from build123d import *

# Parameters (mm, degrees)
SKETCH1_R                = 12.499992756
SKETCH1_R_2              = 4.5
BOSS_EXTRUDE1_DEPTH      = 10
BOSS_EXTRUDE2_DEPTH      = 11
BOSS_EXTRUDE2_DEPTH_BACK = 11
SKETCH7_W                = 11.132946344
SKETCH7_H                = 10.716090789
CUT_EXTRUDE1_DEPTH       = 24
CUT_EXTRUDE2_DEPTH       = 12
SKETCH9_W                = 20
SKETCH9_H                = 14
CUT_EXTRUDE3_DEPTH       = 4
SKETCH11_W               = 3
SKETCH11_H               = 10
CUT_EXTRUDE6_DEPTH       = 29
CUT_EXTRUDE7_DEPTH       = 6
CUT_EXTRUDE8_DEPTH       = 6
SKETCH14_W               = 10
SKETCH14_H               = 16.627390186
CUT_EXTRUDE11_DEPTH      = 1


with BuildPart() as part:
    # Sketch1 → Boss-Extrude1 (new body)
    with BuildSketch(Plane.XY):
        with Locations((-2.359227986, 3.370325694)):
            Circle(SKETCH1_R)
        with Locations((-2.359227986, 3.370325694)):
            Circle(SKETCH1_R_2, mode=Mode.SUBTRACT)
    extrude(amount=BOSS_EXTRUDE1_DEPTH)

    # Sketch2 → Boss-Extrude2 (add, two sides: drawn at the far end of the back side and taken through both)
    with BuildSketch(Plane.XY.offset(5).offset(-BOSS_EXTRUDE2_DEPTH_BACK)):
        with BuildLine():
            Line((-16.466638632, 20.051877412), (-14.375085898, 9.29175702))
            Line((-14.375085898, 9.29175702), (-13.02590258, 9.55401134))
            ThreePointArc((-13.02590258, 9.55401134), (-0.090713324, 14.688621829), (10.07529252, 5.184113893))
            Line((10.07529252, 5.184113893), (10.656286173, 5.533200654))
            Line((10.656286173, 5.533200654), (6.172277384, 28.601437959))
            Line((6.172277384, 28.601437959), (-13.969202109, 48.051877412))
            Line((-13.969202109, 48.051877412), (-42.05953414, 48.051877412))
            ThreePointArc((-42.05953414, 48.051877412), (-44.439585044, 46.878168187), (-44.957305605, 44.275438644))
            Line((-44.957305605, 44.275438644), (-39.806421347, 25.051869783))
            Line((-39.806421347, 25.051869783), (-29.806421347, 25.051869783))
            Line((-29.806421347, 25.051869783), (-28.466638632, 20.051877412))
            Line((-28.466638632, 20.051877412), (-16.466638632, 20.051877412))
        make_face()
    extrude(amount=BOSS_EXTRUDE2_DEPTH + BOSS_EXTRUDE2_DEPTH_BACK)

    # Sketch7 → Cut-Extrude1 (cut)
    with BuildSketch(Plane(origin=(-30.87704133, -8.273389154, 0), x_dir=(0, 0, 1), z_dir=(-0.9659265233912161, -0.2588164434678725, 0))):
        with Locations((5, 44.451666175)):
            Rectangle(SKETCH7_W, SKETCH7_H)
    extrude(amount=-CUT_EXTRUDE1_DEPTH, mode=Mode.SUBTRACT)

    # Sketch8 → Cut-Extrude2 (cut)
    with BuildSketch(Plane(origin=(0, 48.051877412, 0), x_dir=(1, 0, 0), z_dir=(0, 1, 0))):
        Polygon((-42.05953414, 1.356763346), (-42.05953414, -11.393238561), (-40.329492636, -11.393238561), (-40.329492636, -13.893238561), (-30.329492636, -13.893238561), (-30.329492636, -11.393238561), (-18.359521933, -11.393238561), (-18.359521933, 1.356763346), (-30.329492636, 1.356763346), (-30.329492636, 3.856761439), (-40.329492636, 3.856761439), (-40.329492636, 1.356763346), align=None)
    extrude(amount=-CUT_EXTRUDE2_DEPTH, mode=Mode.SUBTRACT)

    # Sketch9 → Cut-Extrude3 (cut)
    with BuildSketch(Plane(origin=(17.270448516, 17.884037296, 0), x_dir=(0.7193391079113861, -0.6946590874877052, 0), z_dir=(0.6946590874877052, 0.7193391079113861, 0))):
        with Locations((-29.428277492, -5)):
            Rectangle(SKETCH9_W, SKETCH9_H)
    extrude(amount=-CUT_EXTRUDE3_DEPTH, mode=Mode.SUBTRACT)

    # Sketch11 → Cut-Extrude6 (cut)
    with BuildSketch(Plane.XY.offset(16)):
        with Locations((-36.641862234, 35.805951308)):
            Rectangle(SKETCH11_W, SKETCH11_H)
    extrude(amount=-CUT_EXTRUDE6_DEPTH, mode=Mode.SUBTRACT)

    # Sketch12 → Cut-Extrude7 (cut)
    with BuildSketch(Plane(origin=(0, 0, -6), x_dir=(-1, 0, 0), z_dir=(0, 0, -1))):
        with BuildLine():
            Line((-11.615804928, 5.778217556), (-10.049600589, 4.877240525))
            ThreePointArc((-10.049600589, 4.877240525), (0.290903423, 13.095654553), (13.015538376, 9.552771876))
            Line((13.015538376, 9.552771876), (14.90302776, 9.185881295))
            Line((14.90302776, 9.185881295), (17.014921429, 20.050637947))
            Line((17.014921429, 20.050637947), (-8.841528869, 20.050637947))
            Line((-8.841528869, 20.050637947), (-11.615804928, 5.778217556))
        make_face()
    extrude(amount=-CUT_EXTRUDE7_DEPTH, mode=Mode.SUBTRACT)

    # Sketch13 → Cut-Extrude8 (cut)
    with BuildSketch(Plane.XY.offset(16)):
        with BuildLine():
            Line((-13.02590258, 9.55401134), (-14.375085898, 9.29175702))
            Line((-14.375085898, 9.29175702), (-16.466638632, 20.051877412))
            Line((-16.466638632, 20.051877412), (7.83414275, 20.051877412))
            Line((7.83414275, 20.051877412), (10.656286173, 5.533200654))
            Line((10.656286173, 5.533200654), (10.07529252, 5.184113893))
            ThreePointArc((10.07529252, 5.184113893), (-0.363045865, 13.248952536), (-13.02590258, 9.55401134))
        make_face()
    extrude(amount=-CUT_EXTRUDE8_DEPTH, mode=Mode.SUBTRACT)

    # Sketch14 → Cut-Extrude11 (cut)
    with BuildSketch(Plane(origin=(11.304697945, 2.197409549, 0), x_dir=(0, 0, -1), z_dir=(0.9816272018550709, 0.1908089006786217, 0))):
        with Locations((-5, 9.874949057)):
            Rectangle(SKETCH14_W, SKETCH14_H)
    extrude(amount=-CUT_EXTRUDE11_DEPTH, mode=Mode.SUBTRACT)


solid = part.part
CAD build for the part. Positions are in the model's coordinates, mm. A direction names the side the tool comes from. Coordinates: 2 decimals unless noted, no trailing zeros. Loops run counter-clockwise (first coordinate to the right, second up) from the corner with the lowest first, then second, coordinate; pieces in that order, holes last. Notation, with made-up numbers: (51.25, -37.5) - (75.25, -37.5) arc R23 cw to (75.25, -9.5) - close; hole circle Ø9 at (87, 51.25). An arc over 180 degrees is marked (long way). Use one line per item in the form item = value. Start each with the question number.
1) Tool access for faces 1 (the face through (-15.436, 14.747, 5.444)), 2 (the face through (-24, 42, 11.393)), 3 (the face through (-42.926, 40.065, 4.922)), 4 (the face through (-3, 9, 0)), 5 (the face through (-38.57, 30.14, 4.92)): list every direction of +Z, -Z, +X, -X, +Y, -Y with a clear straight run to the whole face (end or side of a thin tool).
2) Band-saw the part on B-B (z = 4.5). Give the cut face in (x, y).
3) Band-saw the part on D-D (y = 26). Give the cut face in (x, z), and give its area (3 significant figures).
4) Band-saw the part on A-A (x = -2). Give the cut face in (y, z).
5) Flat gauge pins, fed straight in: pin 1 (6 mm diameter, centred on x = -38, y = 37, fed in from -Z); pin 2 (2.5 mm diameter, centred on x = -36.5, z = 3, fed in from +Y); pin 3 (2.5 mm diameter, centred on x = -36.5, z = 15, fed in from -Y); pin 4 (1.5 mm diameter, centred on y = 1.5, z = 9, fed in from -X). Where does each tip first touch, or does it go through?
6) Two-plate mould, pull along X, no slides. Class faces 6 (the face through (-30.329, 42, 13)), 7 (the face through (-12.462, 43.855, 5.098)), 8 (the face through (-18.09, 36.73, 4.92)): +X half, -X half, draft (parallel to the pull), parting line (faces both ways), or undercut.
7) Band-saw the part on C-C (x = -21). Give the cut face in (y, z).
8) Drill centre lines: L1, parallel to Z at x = -27.5, y = 46; L2, parallel to Z at x = -6, y = 36; L3, parallel to Y at x = -38.5, z = -4.75. Where is each one in solid material? Low to high. Write a range as from..to.
Check values:
q1.face_1 = +Z, -Z, -X
q1.face_2 = +Y
q1.face_3 = -Y
q1.face_4 = -Z, +X, -X, -Y
q1.face_5 = -X, +Y
q2.outline = (-44.96, 44.28) - (-43.77, 39.84) - (-42.06, 40.3) - (-42.06, 48.05) arc R3 ccw to start; (-41, 29.49) - (-39.81, 25.05) - (-29.81, 25.05) - (-28.47, 20.05) - (-16.47, 20.05) - (-14.38, 9.29) - (-13.25, 9.51) arc R12.5 ccw (long way) to (10.14, 3.56) - (10.03, 3.54) - (6.85, 19.86) - (7.83, 20.05) - (6.17, 28.6) - (3.29, 31.38) - (0.52, 28.5) - (-13.87, 42.4) - (-11.09, 45.27) - (-13.97, 48.05) - (-18.36, 48.05) - (-18.36, 37.74) - (-17.81, 35.7) - (-35.14, 31.06) - (-35.14, 30.81) - (-36.08, 30.81) - close; hole circle Ø9 at (-2.36, 3.37)
q3.outline = (-40.06, -6) - (6.68, -6) - (6.68, 16) - (-40.06, 16) - close
q3.area = 1,030 mm2
q4.outline = (-9.12, 0) - (-1.12, 0) - (-1.12, 10) - (-9.12, 10) - close; (7.86, 0) - (20.05, 0) - (20.05, -6) - (36.49, -6) - (36.49, -2) - (30.93, -2) - (30.93, 12) - (36.49, 12) - (36.49, 16) - (20.05, 16) - (20.05, 10) - (7.86, 10) - close
q5.pin_1 = -6
q5.pin_2 = 30.81
q5.pin_3 = 25.05
q5.pin_4 = -14.81
q6.face_6 = undercut
q6.face_7 = +X half
q6.face_8 = -X half
q7.outline = (20.05, -6) - (48.05, -6) - (48.05, -1.36) - (36.05, -1.36) - (36.05, -0.57) - (34.85, -0.57) - (34.85, 10.57) - (36.05, 10.57) - (36.05, 11.39) - (48.05, 11.39) - (48.05, 16) - (20.05, 16) - close
q8.L1 = -6..-1.36, 11.39..16
q8.L2 = -6..-2, 12..16
q8.L3 = 25.05..48.05
